Build history of the part. All positions in model axes, mm. A direction names the side the tool comes from. Give positions to 0.01 mm unless a question says otherwise; leave off trailing zeros. Order: outer loops, then holes, each group sorted by start corner. A loop starts at its lowest first (then second) coordinate and runs counter-clockwise, first axis right, second up. Notation, with made-up numbers: M 10.5,47 L 20.5,47 A6 cw 20.5,58 Z; hole C -28,84.5 d11. An arc over 180 degrees is marked long. One line per item, written item: value.
from build123d import *

# Parameters (mm, degrees)
BASE_FLANGE1_DEPTH   = 3.175
M6_CLEARANCE_HOLE1_D = 6.6
FILLET1_R            = 2.54


# Sheet-metal steps are written as plain solids
with BuildPart() as part:
    # Sketch1 → Base-Flange1 (new body)
    with BuildSketch(Plane.XY):
        Polygon((63.66772505, -78.480441727), (47.205847983, -62.123600001), (-25.819152017, -62.123600001), (-25.819152017, -78.501600001), (40.496105752, -78.501600001), (47.28972505, -85.338441727), (47.28972505, -101.340441727), (63.66772505, -101.340441727), align=None)
    extrude(amount=-BASE_FLANGE1_DEPTH)

    # M6 Clearance Hole1 (through all)
    with Locations(Plane.XY):
        with Locations((56.565919048, -91.535610498), (-17.0119, -70.312600001)):
            Hole(M6_CLEARANCE_HOLE1_D / 2)

    # Fillet1
    fillet1_edges = [part.edges().sort_by_distance(p)[0] for p in [
        (-25.819152017, -62.123600001, -1.5875),
        (47.205847983, -62.123600001, -1.5875),
        (63.66772505, -78.480441727, -1.5875),
        (63.66772505, -101.340441727, -1.5875),
        (47.28972505, -101.340441727, -1.5875),
        (47.28972505, -85.338441727, -1.5875),
        (40.496105752, -78.501600001, -1.5875),
        (-25.819152017, -78.501600001, -1.5875),
    ]]
    fillet(fillet1_edges, radius=FILLET1_R)


solid = part.part
1) Saw through at D-D, the plane y = -97. Write the cut outline in (x, z) (3 decimals), then the cut area to 3 significant figures.
Check values:
outline: M 47.29,-3.175 L 63.668,-3.175 L 63.668,0 L 47.29,0 Z
area: 52.0 mm^2
2) Saw through at B-B, the plane z = -0.7. Write the cut outline in (x, y).
Check values:
outline: M -25.82,-75.96 A2.54 ccw -23.28,-78.5 L 39.44,-78.5 A2.54 cw 41.24,-79.25 L 46.55,-84.6 A2.54 cw 47.29,-86.39 L 47.29,-98.8 A2.54 ccw 49.83,-101.34 L 61.13,-101.34 A2.54 ccw 63.67,-98.8 L 63.67,-79.54 A2.54 ccw 62.92,-77.74 L 47.95,-62.86 A2.54 ccw 46.16,-62.12 L -23.28,-62.12 A2.54 ccw -25.82,-64.66 Z; hole C -17.01,-70.31 d6.6; hole C 56.57,-91.54 d6.6
3) Saw through at C-C, the plane y = -72. Write the cut outline in (x, z) (3 decimals).
Check values:
outline: M -25.819,-3.175 L -19.848,-3.175 L -19.848,0 L -25.819,0 Z; M -14.176,-3.175 L 57.146,-3.175 L 57.146,0 L -14.176,0 Z
4) Saw through at A-A, the plane x = -19. Write the cut outline in (y, z) (1 decimal), then the cut area to 3 significant figures.
Check values:
outline: M -78.5,-3.2 L -72.9,-3.2 L -72.9,0 L -78.5,0 Z; M -67.7,-3.2 L -62.1,-3.2 L -62.1,0 L -67.7,0 Z
area: 35.3 mm^2
5) Mould opens along Y. For faces 3 (the face through (53.42, -90.54, -1.61)), 4 (the face through (62.94, -100.58, -1.61)), 5 (the face through (18, -73, 0)) say: released by +Y, released by -Y, zero draft, split by the parting line, or undercut.
Check values:
face 3: undercut
face 4: released by -Y
face 5: zero draft
6) Pin check, flat tips, straight feed: pin 1 (1 mm diameter, centred on x = 15, y = -76.5, fed in from +Z); pin 2 (1 mm diameter, centred on x = 1.5, z = -0.5, fed in from -Y); pin 3 (1.6 mm diameter, centred on y = -90.5, z = -1.5, fed in from -X). Stop position of each tip, or through.
Check values:
pin 1: z = 0
pin 2: y = -78.5
pin 3: x = 47.29
7) Drill centre lines: probe 1 along Y at (x, z) = (4, -2.65); probe 2 along X at (y, z) = (-72, -2.2); probe 3 along X at (y, z) = (-71.5, -2.3). Where is each one in solid material? Low to high. Write a range as from..to.
Check values:
probe 1: -78.5..-62.12
probe 2: -25.82..-19.85, -14.18..57.15
probe 3: -25.82..-20.09, -13.93..56.64
8) Tool access for faces 1 (the face through (47.29, -93, -2)), 2 (the face through (47.14, -62.32, -1.61)): list every direction of +Z, -Z, +X, -X, +Y, -Y with a clear straight run to the whole face (end or side of a thin tool).
Check values:
face 1: +Z, -Z, -X, -Y
face 2: +Z, -Z, +X, +Y
